```python
from build123d import *

# Parameters (mm, degrees)
BOSS_EXTRU_1_DEPTH                              = 12
CHAMBRAGE_POUR_VIS_T_TE_CYLINDRIQUE_D           = 2.5
CHAMBRAGE_POUR_VIS_T_TE_CYLINDRIQUE_CBORE_D     = 4.5
CHAMBRAGE_POUR_VIS_T_TE_CYLINDRIQUE_CBORE_DEPTH = 10
ESQUISSE12_R                                    = 8
ENL_V_MAT_EXTRU_1_DEPTH                         = 7
ESQUISSE14_R                                    = 2
ENL_V_MAT_EXTRU_2_DEPTH                         = 10
ESQUISSE15_R                                    = 4.25
ENL_V_MAT_EXTRU_3_DEPTH                         = 20.927995444


with BuildPart() as part:
    # Esquisse1 → Boss.-Extru.1 (new body)
    with BuildSketch(Plane(origin=(0, 0, 0), x_dir=(1, 0, 0), z_dir=(0, 1, 0))):
        with BuildLine():
            Line((6.025985397, 9.5), (-6.025985397, 9.5))
            ThreePointArc((-6.025985397, 9.5), (0, -11.25), (6.025985397, 9.5))
        make_face()
    extrude(amount=BOSS_EXTRU_1_DEPTH)

    # Chambrage pour vis à tête cylindrique à 6 pans creux (ou vis CHC) M21 (through all)
    with Locations(Plane(origin=(0, 12, 0), x_dir=(1, 0, 0), z_dir=(0, 1, 0))):
        with Locations((8, 0), (0, -8), (-8, 0)):
            CounterBoreHole(CHAMBRAGE_POUR_VIS_T_TE_CYLINDRIQUE_D / 2, CHAMBRAGE_POUR_VIS_T_TE_CYLINDRIQUE_CBORE_D / 2, CHAMBRAGE_POUR_VIS_T_TE_CYLINDRIQUE_CBORE_DEPTH)

    # Esquisse12 → Enlèv. mat.-Extru.1 (cut)
    with BuildSketch(Plane(origin=(0, 12, 0), x_dir=(1, 0, 0), z_dir=(0, 1, 0))):
        Circle(ESQUISSE12_R)
    extrude(amount=-ENL_V_MAT_EXTRU_1_DEPTH, mode=Mode.SUBTRACT)

    # Esquisse14 → Enlèv. mat.-Extru.2 (cut)
    with BuildSketch(Plane(origin=(0, 0, -9.5), x_dir=(-1, 0, 0), z_dir=(0, 0, -1))):
        with Locations((0, 9)):
            Circle(ESQUISSE14_R)
    extrude(amount=-ENL_V_MAT_EXTRU_2_DEPTH, mode=Mode.SUBTRACT)

    # Esquisse15 → Enlèv. mat.-Extru.3 (cut, through all)
    with BuildSketch(Plane.XZ):
        with Locations(Location((0, 0, 0), (0, 0, 270))):
            Circle(ESQUISSE15_R)
    extrude(amount=-ENL_V_MAT_EXTRU_3_DEPTH, mode=Mode.SUBTRACT)


solid = part.part
```
Build history of the part. All positions in model axes, mm. A direction names the side the tool comes from. Give positions to 0.01 mm unless a question says otherwise; leave off trailing zeros. Order: outer loops, then holes, each group sorted by start corner. A loop starts at its lowest first (then second) coordinate and runs counter-clockwise, first axis right, second up. Notation, with made-up numbers: M 63.5,6.5 L 106.5,6.5 A23 ccw 106.5,31.5 Z; hole C -33,84 d5. An arc over 180 degrees is marked long. Return JSON: item names as keys, results as strings.
Q1. Band-saw the part on A-A (x = 0). Give the cut face in (y, z), then the cut area to 4 significant figures.
Answer list:
{"outline": "M 0,-9.5 L 7,-9.5 L 7,-8 L 5,-8 L 5,-4.25 L 0,-4.25 Z; M 0,4.25 L 5,4.25 L 5,5.75 L 2,5.75 L 2,6.75 L 0,6.75 Z; M 0,9.25 L 2,9.25 L 2,10.25 L 12,10.25 L 12,11.25 L 0,11.25 Z; M 11,-9.5 L 12,-9.5 L 12,-8 L 11,-8 Z", "area": "54.25 mm^2"}
Q2. Two-plate mould, pull along Z, no slides. Class faces 1 (the face through (0, 6, -9.5)), 2 (the face through (2.4, 8.55, -7.63)), 3 (the face through (-0.406, 5.916, 11.243)), 4 (the face through (-3, 12, 8)): pulls with the +Z half, pulls with the -Z half, needs draft (parallel to the pull), parting line crosses it, or undercut.
Answer list:
{"face 1": "pulls with the -Z half", "face 2": "undercut", "face 3": "parting line crosses it", "face 4": "needs draft"}
Q3. Wall check: probe 1 along Y at (x, z) = (0, -8.5); probe 2 along Y at (x, z) = (-2.5, 4.75); probe 3 along X at (y, z) = (9.5, -2). Give the ranges that are in metal, low to high. Write a range as from..to.
Answer list:
{"probe 1": "y = 0..7, 11..12", "probe 2": "y = 0..5", "probe 3": "x = -11.07..-9.03, 9.03..11.07"}
Q4. Band-saw the part on C-C (x = 8.5). Give the cut face in (y, z).
Answer list:
{"outline": "M 0,-7.37 L 12,-7.37 L 12,-2.19 L 2,-2.19 L 2,-1.15 L 0,-1.15 Z; M 0,1.15 L 2,1.15 L 2,2.19 L 12,2.19 L 12,7.37 L 0,7.37 Z"}
Q5. Band-saw the part on D-D (y = 1). Give the cut face in (x, z).
Answer list:
{"outline": "M -6.03,-9.5 L 6.03,-9.5 A11.25 ccw long Z; hole C -8,0 d2.5; hole C 0,0 d8.5; hole C 0,8 d2.5; hole C 8,0 d2.5"}
Q6. Flat gauge pins, fed straight in: pin 1 (2 mm diameter, centred on x = 7, z = 1, fed in from +Y); pin 2 (1.5 mm diameter, centred on x = -9, y = 10, fed in from +Z); pin 3 (3.5 mm diameter, centred on x = -8, z = 0, fed in from +Y). Where does each tip first touch, or does it go through?
Answer list:
{"pin 1": "stops at y = 5", "pin 2": "stops at z = 7.65", "pin 3": "stops at y = 2"}
Q7. 3-axis set-ups, long thin cutter, end or side, ignore diameter. For faces 5 (the face through (-6.75, 0.99, -0.05)), 6 (the face through (1, 2, 9)), 7 (the face through (-0.923, 7.226, -8.632)): which of +Z, -Z, +X, -X, +Y, -Y reach the whole face in a straight line?
Answer list:
{"face 5": "+Y, -Y", "face 6": "+Y", "face 7": "-Z"}
Q8. Band-saw the part on B-B (z = 8). Give the cut face in (x, y).
Answer list:
{"outline": "M -7.91,0 L -1.25,0 L -1.25,2 L -2.25,2 L -2.25,12 L -7.91,12 Z; M 1.25,0 L 7.91,0 L 7.91,12 L 2.25,12 L 2.25,2 L 1.25,2 Z"}
